```python
from build123d import *

# Parameters (mm, degrees)
SKETCH_1_W              = 120
SKETCH_1_H              = 80
EXTRUDE_1_DEPTH         = 6
SKETCH_3_R              = 2.05
CUT_EXTRUDE_4_1_1_DEPTH = 5
SKETCH_4_R              = 2.05
CUT_EXTRUDE_4_1_2_DEPTH = 5
SKETCH_5_R              = 4
CUT_EXTRUDE_3_DEPTH     = 3
SKETCH_6_R              = 7.5
CUT_EXTRUDE_4_DEPTH     = 10


with BuildPart() as part:
    # 草图1 → 凸台-拉伸1 (new body)
    with BuildSketch(Plane(origin=(0, 0, 0), x_dir=(1, 0, 0), z_dir=(0, 1, 0))):
        Rectangle(SKETCH_1_W, SKETCH_1_H)
    extrude(amount=EXTRUDE_1_DEPTH)

    # 草图3 → φ4.1孔1 (cut)
    with BuildSketch(Plane(origin=(0, 6, 0), x_dir=(1, 0, 0), z_dir=(0, 1, 0))):
        with Locations(Location((0, -20, 0), (0, 0, 270))):
            Circle(SKETCH_3_R)
        with Locations(Location((-17.320508076, 10, 0), (0, 0, 270))):
            Circle(SKETCH_3_R)
        with Locations(Location((17.320508076, 10, 0), (0, 0, 270))):
            Circle(SKETCH_3_R)
    extrude(amount=-CUT_EXTRUDE_4_1_1_DEPTH, mode=Mode.SUBTRACT)

    # 草图4 → φ4.1孔2 (cut)
    with BuildSketch(Plane.XZ):
        with Locations(Location((-16.454482672, 9.5, 0), (0, 0, 270))):
            Circle(SKETCH_4_R)
        with Locations(Location((16.454482672, 9.5, 0), (0, 0, 270))):
            Circle(SKETCH_4_R)
        with Locations(Location((0, -19, 0), (0, 0, 270))):
            Circle(SKETCH_4_R)
    extrude(amount=-CUT_EXTRUDE_4_1_2_DEPTH, mode=Mode.SUBTRACT)

    # 草图5 → 切除-拉伸3 (cut)
    with BuildSketch(Plane.XZ):
        with Locations(Location((-16.454482672, 9.5, 0), (0, 0, 270))):
            Circle(SKETCH_5_R)
        with Locations(Location((16.454482672, 9.5, 0), (0, 0, 270))):
            Circle(SKETCH_5_R)
        with Locations(Location((0, -19, 0), (0, 0, 270))):
            Circle(SKETCH_5_R)
    extrude(amount=-CUT_EXTRUDE_3_DEPTH, mode=Mode.SUBTRACT)

    # 草图6 → 切除-拉伸4 (cut)
    with BuildSketch(Plane.XZ):
        with Locations(Location((0, 0, 0), (0, 0, 270))):
            Circle(SKETCH_6_R)
    extrude(amount=-CUT_EXTRUDE_4_DEPTH, mode=Mode.SUBTRACT)


solid = part.part
```
The model under review builds one solid part; all positions refer to its coordinate system, in mm. A direction names the side the tool comes from. Give positions to 0.01 mm unless a question says otherwise; leave off trailing zeros. Write each loop counter-clockwise with the first axis right and the second up, starting at its lowest first coordinate (ties: lowest second). Pieces come first, ordered by that corner, then holes.
(1) The part is to be moulded in two halves that separate along X. For faces 1 (the flat face through (60, 3, 1)), 2 (the flat face through (-1, 6, -9)), 3 (the cylindrical face through (-18.888, 1.479, 12.674)), say which applies: released by +X, released by -X, zero draft, split by the parting line, or undercut.
(2) For P1, Ø2.5, axis at x = -17.5, z = 9.5, coming from the -Y side; P2, Ø4.5, axis at x = 17.32, z = -10, coming from the -Y side; P3, Ø2, axis at x = -16.5, z = 9, coming from the -Y side; P4, Ø3.5, axis at x = -17.32, z = -10, coming from the +Y side, all flat-tipped, find the tip position at first contact; note any pin that passes through.
(3) Consider section C-C, the plane z = 9.5. Give the boundary of the cut face in (x, y), and give its area (3 significant figures).
(4) Consider section A-A, the plane x = 0. Give the boundary of the cut face in (y, z).
(5) Tool access review of faces 4 (the cylindrical face through (18.706, 3.535, -11.511)), 5 (the flat face through (-18.2, 3, 7.8)), 6 (the flat face through (-1, 3, -40)): name each direction out of +Z, -Z, +X, -X, +Y, -Y from which nothing blocks a thin tool from reaching the whole face with its end or side.
(6) Consider section B-B, the plane z = -10. Give the boundary of the cut face in (x, y), and give its area (3 significant figures).
(7) Consider section D-D, the plane z = 20. Give the boundary of the cut face in (x, y).
(8) To check wall thickness, follow L1, parallel to X at y = 2.1, z = 9.5; L2, parallel to X at y = 4.5, z = 9.5; L3, parallel to X at y = 3.95, z = 20. State the ranges of each line that lie inside material, in increasing order.
Returned:
1. face 1: released by +X
1. face 2: zero draft
1. face 3: undercut
2. P1: stops at y = 3
2. P2: stops at y = 0
2. P3: stops at y = 5
2. P4: stops at y = 1
3. outline: (-60, 0) - (-20.45, 0) - (-20.45, 3) - (-18.5, 3) - (-18.5, 5) - (-14.4, 5) - (-14.4, 3) - (-12.45, 3) - (-12.45, 0) - (12.45, 0) - (12.45, 3) - (14.4, 3) - (14.4, 5) - (18.5, 5) - (18.5, 3) - (20.45, 3) - (20.45, 0) - (60, 0) - (60, 6) - (-60, 6) - close
3. area: 656 mm2
4. outline: (0, -40) - (6, -40) - (6, -7.5) - (0, -7.5) - (0, -15) - (3, -15) - (3, -16.95) - (5, -16.95) - (5, -21.05) - (3, -21.05) - (3, -23) - (0, -23) - close; (0, 7.5) - (6, 7.5) - (6, 17.95) - (1, 17.95) - (1, 22.05) - (6, 22.05) - (6, 40) - (0, 40) - close
5. face 4: +Y
5. face 5: -Y
5. face 6: -Z, +X, -X, +Y, -Y
6. outline: (-60, 0) - (60, 0) - (60, 6) - (19.37, 6) - (19.37, 1) - (15.27, 1) - (15.27, 6) - (-15.27, 6) - (-15.27, 1) - (-19.37, 1) - (-19.37, 6) - (-60, 6) - close
6. area: 679 mm2
7. outline: (-60, 0) - (60, 0) - (60, 6) - (2.05, 6) - (2.05, 1) - (-2.05, 1) - (-2.05, 6) - (-60, 6) - close
8. L1: x = -60 to -20.45, -12.45 to 12.45, 20.45 to 60
8. L2: x = -60 to -18.5, -14.4 to 14.4, 18.5 to 60
8. L3: x = -60 to -2.05, 2.05 to 60
